```python
from build123d import *

# Parameters (mm, degrees)
BOSS_EXTRUDE1_DEPTH = 150


with BuildPart() as part:
    # Sketch1 → Boss-Extrude1 (new, symmetric)
    with BuildSketch(Plane.XY):
        with BuildLine():
            Line((0, -50), (1300, -50))
            ThreePointArc((1300, -50), (1350, 0), (1300, 50))
            Line((1300, 50), (0, 50))
            ThreePointArc((0, 50), (-50, 0), (0, -50))
        make_face()
        with BuildLine():
            ThreePointArc((0, 44), (-44, 0), (0, -44))
            Line((0, -44), (1300, -44))
            ThreePointArc((1300, -44), (1344, 0), (1300, 44))
            Line((1300, 44), (0, 44))
        make_face(mode=Mode.SUBTRACT)
    extrude(amount=BOSS_EXTRUDE1_DEPTH, both=True)


solid = part.part
```
For this review, take the finished solid that the model builds, in its own axes (mm). A direction names the side the tool comes from. Coordinates: 2 decimals unless noted, no trailing zeros. Order: outer loops, then holes, each group sorted by start corner. A loop starts at its lowest first (then second) coordinate and runs counter-clockwise, first axis right, second up. Notation, with made-up numbers: (64, -26) -> (75, -26) arc R26 cw to (75, -8) -> close; hole circle Ø3 at (-9, 41.5). An arc over 180 degrees is marked (long way). Answer as CSV lines item,"result".
Q1. Draft analysis for pull direction X (two halves, no side actions). For faces 1 (the face through (-49.988, 1.099, 2.1)), 2 (the face through (1349.988, -1.099, 2.1)), 3 (the face through (641, -50, 2)), 4 (the face through (659, 44, 2)), state which applies: released by +X, released by -X, zero draft, split by the parting line, or undercut.
Model answer:
face 1,"released by -X"
face 2,"released by +X"
face 3,"zero draft"
face 4,"undercut"
Q2. We need section C-C (z = 37). State the section outline as (x, y) points, plus the area to 3 significant figures.
Model answer:
outline,"(0, -50) -> (1300, -50) arc R50 ccw to (1300, 50) -> (0, 50) arc R50 ccw to start; hole (0, -44) -> (1300, -44) arc R44 ccw to (1300, 44) -> (0, 44) arc R44 ccw to start"
area,"17,400 mm2"
Q3. We need section A-A (x = 344.5). State the section outline as (y, z) points, plus the area to 3 significant figures.
Model answer:
outline,"(-50, -150) -> (-44, -150) -> (-44, 150) -> (-50, 150) -> close; (44, -150) -> (50, -150) -> (50, 150) -> (44, 150) -> close"
area,"3,600 mm2"
Q4. For faces 5 (the face through (1343.99, -0.97, 2.1)), 6 (the face through (647, 45, 150)), list the 3-axis set-ups (+Z, -Z, +X, -X, +Y, -Y) from which the entire face can be reached by the end or side of a thin tool; tool diameter is ignored.
Model answer:
face 5,"+Z, -Z"
face 6,"+Z, +X, -X, +Y, -Y"
Q5. We need section B-B (y = 0). State the section outline as (x, z) points, plus the area to 3 significant figures.
Model answer:
outline,"(-50, -150) -> (-44, -150) -> (-44, 150) -> (-50, 150) -> close; (1344, -150) -> (1350, -150) -> (1350, 150) -> (1344, 150) -> close"
area,"3,600 mm2"
Q6. Wall thickness on line 1 along Y through (x, z) = (850, -118.5); line 2 along X through (y, z) = (-2, 95.5); line 3 along X through (y, z) = (-3.5, -39.5): over which ranges is each line inside the solid? List them lowest first. Write a range as [from, to].
Model answer:
line 1,"y = [-50, -44], [44, 50]"
line 2,"x = [-49.96, -43.95], [1343.95, 1349.96]"
line 3,"x = [-49.88, -43.86], [1343.86, 1349.88]"
Q7. Clearance check with flat-ended pins moving along their axes: pin 1 Ø1 at (y, z) = (-16, -99) entering from +X; pin 2 Ø1.5 at (y, z) = (-40, -47.5) entering from +X. State where each tip first meets the part, or that it passes through.
Model answer:
pin 1,"stops at x = 1347.54"
pin 2,"stops at x = 1330.97"
